The listing builds one solid part. Answer for the finished solid, in the listing's coordinates (mm). Coordinates: 2 decimals unless noted, no trailing zeros. Order: outer loops, then holes, each group sorted by start corner. A loop starts at its lowest first (then second) coordinate and runs counter-clockwise, first axis right, second up. Notation, with made-up numbers: (-12.75, 55.5) -> (33.25, 55.5) arc R23 ccw to (33.25, 69.5) -> close; hole circle Ø1 at (70, 13.25). An arc over 180 degrees is marked (long way). Write item = value, one per line.
from build123d import *

# Parameters (mm, degrees)
SKETCH_1_R             = 6
EXTRUDE_1_DEPTH        = 3
SKETCH_2_R             = 6
EXTRUDE_2_DEPTH        = 13
HOLE_WIZARD_M6_1_D     = 5
HOLE_WIZARD_M6_1_DEPTH = 12
HOLE_WIZARD_M6_1_TIP   = 1.502151548
SKETCH_6_R             = 3
CUT_EXTRUDE_1_DEPTH    = 10


with BuildPart() as part:
    # 草图1 → 凸台-拉伸1 (new body)
    with BuildSketch(Plane(origin=(0, 0, 0), x_dir=(1, 0, 0), z_dir=(0, 1, 0))):
        with Locations((-13.5, 0)):
            Circle(SKETCH_1_R)
        with BuildLine():
            Line((13.5, 6), (-13.5, 6))
            ThreePointArc((-13.5, 6), (-9.257359313, 4.242640687), (-7.5, 0))
            ThreePointArc((-7.5, 0), (-9.257359313, -4.242640687), (-13.5, -6))
            Line((-13.5, -6), (13.5, -6))
            ThreePointArc((13.5, -6), (7.5, 0), (13.5, 6))
        make_face()
        with Locations((13.5, 0)):
            Circle(SKETCH_1_R)
        with BuildLine():
            Line((-13.5, -6), (-13.5, 6))
            ThreePointArc((-13.5, 6), (-19.5, 0), (-13.5, -6))
        make_face()
        with BuildLine():
            ThreePointArc((19.5, 0), (17.742640687, 4.242640687), (13.5, 6))
            Line((13.5, 6), (13.5, -6))
            ThreePointArc((13.5, -6), (17.742640687, -4.242640687), (19.5, 0))
        make_face()
    extrude(amount=EXTRUDE_1_DEPTH)

    # 草图2 → 凸台-拉伸2 (add)
    with BuildSketch(Plane(origin=(0, 3, 0), x_dir=(1, 0, 0), z_dir=(0, 1, 0))):
        Circle(SKETCH_2_R)
    extrude(amount=EXTRUDE_2_DEPTH)

    # M6 螺纹孔1
    with Locations(Plane(origin=(0, 16, 0), x_dir=(1, 0, 0), z_dir=(0, 1, 0))):
        with Locations((0, 0)):
            Hole(HOLE_WIZARD_M6_1_D / 2, depth=HOLE_WIZARD_M6_1_DEPTH)
            with Locations((0, 0, -(HOLE_WIZARD_M6_1_DEPTH + HOLE_WIZARD_M6_1_TIP / 2))):  # 118° drill point
                Cone(0, HOLE_WIZARD_M6_1_D / 2, HOLE_WIZARD_M6_1_TIP, mode=Mode.SUBTRACT)

    # 草图6 → 切除-拉伸1 (cut)
    with BuildSketch(Plane(origin=(0, 3, 0), x_dir=(1, 0, 0), z_dir=(0, 1, 0))):
        with Locations((-13.5, 0)):
            Circle(SKETCH_6_R)
        with Locations((13.5, 0)):
            Circle(SKETCH_6_R)
    extrude(amount=-CUT_EXTRUDE_1_DEPTH, mode=Mode.SUBTRACT)


solid = part.part
Q1. Section A-A, the plane x = 12.5 is taken. Give the vertices of the cut face in (y, z), plus the area to 3 significant figures.
The answers:
outline = (0, -6) -> (3, -6) -> (3, -2.83) -> (0, -2.83) -> close; (0, 2.83) -> (3, 2.83) -> (3, 6) -> (0, 6) -> close
area = 19.0 mm2
Q2. Find the intervals of material crossed by line 1 along X through (y, z) = (2.1, 0); line 2 along Z through (x, y) = (13.5, 1.85); line 3 along Z through (x, y) = (0, 12.75), in increasing order.
The answers:
line_1 = -19.5 to -16.5, -10.5 to 10.5, 16.5 to 19.5
line_2 = -6 to -3, 3 to 6
line_3 = -6 to -2.5, 2.5 to 6
Q3. Section B-B, the plane y = 9.25 is taken. Give the vertices of the cut face in (x, z).
The answers:
outline = circle Ø12 at (0, 0); hole circle Ø5 at (0, 0)
Q4. Section C-C, the plane x = -5 is taken. Give the vertices of the cut face in (y, z), plus the area to 3 significant figures.
The answers:
outline = (0, -6) -> (3, -6) -> (3, -3.32) -> (16, -3.32) -> (16, 3.32) -> (3, 3.32) -> (3, 6) -> (0, 6) -> close
area = 122 mm2
Q5. Section D-D, the plane z = -3.5 is taken. Give the vertices of the cut face in (x, y), plus the area to 3 significant figures.
The answers:
outline = (-18.37, 0) -> (18.37, 0) -> (18.37, 3) -> (4.87, 3) -> (4.87, 16) -> (-4.87, 16) -> (-4.87, 3) -> (-18.37, 3) -> close
area = 237 mm2
Q6. The mould has two halves that part along X. Classify faces 1 (the face through (19.5, 1.5, 0.1)), 2 (the face through (-6, 9, 0)), 3 (the face through (0, 1, -6)), 4 (the face through (0.54, 9.92, 2.44)): released by +X, released by -X, zero draft, split by the parting line, or undercut.
The answers:
face_1 = released by +X
face_2 = split by the parting line
face_3 = zero draft
face_4 = undercut
Q7. Each of these flat-tipped pins is pushed along its axis until it touches: pin 1 Ø6 at (x, z) = (-8, -2) entering from +Y; pin 2 Ø4 at (y, z) = (4.5, -4) entering from -X; pin 3 Ø4 at (y, z) = (11, -4.5) entering from +X; pin 4 Ø2 at (y, z) = (2.5, -2) entering from +X. Where does it stop, or does it pass through?
The answers:
pin_1 = 16
pin_2 = -18.87
pin_3 = 5.45
pin_4 = 19.42
